from build123d import *

# Parameters (mm, degrees)
SKETCH1_R           = 6
SKETCH1_R_2         = 4.5
BOSS_EXTRUDE1_DEPTH = 0.5
CUT_EXTRUDE1_START  = -0.5
CUT_EXTRUDE1_DEPTH  = 0.5
FILLET1_R           = 1


with BuildPart() as part:
    # Sketch1 → Boss-Extrude1 (new body)
    with BuildSketch(Plane.XY):
        Circle(SKETCH1_R)
        Circle(SKETCH1_R_2, mode=Mode.SUBTRACT)
    extrude(amount=BOSS_EXTRUDE1_DEPTH)

    # Sketch2 → Cut-Extrude1 (cut)
    with BuildSketch(Plane.XY.offset(0.5).offset(CUT_EXTRUDE1_START)):
        with BuildLine():
            Line((5.637224766, 2.054676846), (4.227918574, 1.541007634))
            ThreePointArc((4.227918574, 1.541007634), (4.431457637, 0.782421375), (4.5, 0))
            ThreePointArc((4.5, 0), (4.431457637, -0.782421375), (4.227918574, -1.541007634))
            Line((4.227918574, -1.541007634), (5.637224766, -2.054676846))
            ThreePointArc((5.637224766, -2.054676846), (5.908610183, -1.0432285), (6, 0))
            ThreePointArc((6, 0), (5.908610183, 1.0432285), (5.637224766, 2.054676846))
        make_face()
    extrude(amount=CUT_EXTRUDE1_DEPTH, mode=Mode.SUBTRACT)

    # Fillet1
    # the kernel refuses this fillet: 1 mm, written as the material it takes off along each edge
    with BuildSketch(Plane(origin=(4.227918574, -1.541007634, -2.270817283), x_dir=(0.9395374609645726, -0.3424461409393371, 0), z_dir=(0, 0, 1))) as fillet1_piece_1:
        with BuildLine():
            CenterArc((0.908326913, -1), FILLET1_R, 90, 79.524318304)
            ThreePointArc((-0.075005253, -0.818181818), (-0.018790545, -0.410806303), (0, 0))
            Line((0, 0), (0.908326913, 0))
        make_face()
    extrude(amount=5.041634566, mode=Mode.SUBTRACT)
    with BuildSketch(Plane(origin=(5.637224766, -2.054676846, -3.01526886), x_dir=(-0.4351439810441928, -0.9003608808477915, 0), z_dir=(0, 0, 1))) as fillet1_piece_2:
        with BuildLine():
            CenterArc((1.105598582, -0.994936153), FILLET1_R, 84.231520484, 101.536959033)
            Line((0.110662429, -1.095445115), (0, 0))
            ThreePointArc((0, 0), (0.603053772, 0.030383082), (1.206107544, 0))
        make_face()
    extrude(amount=6.53053772, mode=Mode.SUBTRACT)
    with BuildSketch(Plane(origin=(4.227918574, 1.541007634, -2.270817283), x_dir=(0.9395374609645728, 0.3424461409393367, 0), z_dir=(0, 0, 1))) as fillet1_piece_3:
        with BuildLine():
            CenterArc((0.908326913, 1), FILLET1_R, 190.475681696, 79.524318304)
            ThreePointArc((-0.075005253, 0.818181818), (-0.018790545, 0.410806303), (0, 0))
            Line((0, 0), (0.908326913, 0))
        make_face()
    extrude(amount=5.041634566, mode=Mode.SUBTRACT)
    with BuildSketch(Plane(origin=(5.637224766, 2.054676846, -3.01526886), x_dir=(-0.43514398104419194, 0.9003608808477921, 0), z_dir=(0, 0, 1))) as fillet1_piece_4:
        with BuildLine():
            CenterArc((1.105598582, 0.994936153), FILLET1_R, 174.231520484, 101.536959033)
            Line((0.110662429, 1.095445115), (0, 0))
            ThreePointArc((0, 0), (0.603053772, -0.030383082), (1.206107544, 0))
        make_face()
    extrude(amount=6.53053772, mode=Mode.SUBTRACT)


solid = part.part
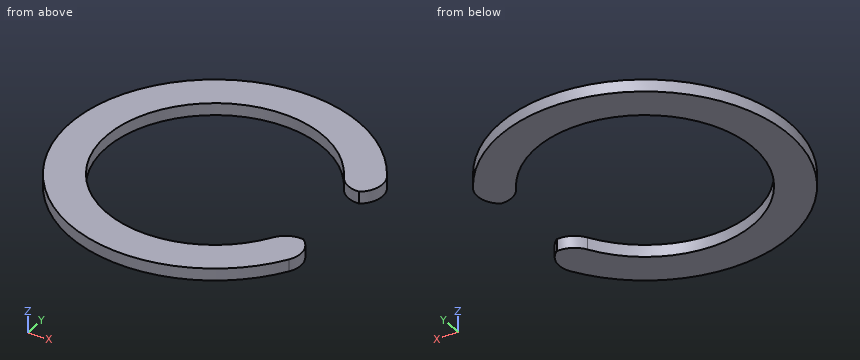
Source: CAD feature listing. Evaluate the final solid. Frame: model axes, mm. Give positions to 0.01 mm unless a question says otherwise; leave off trailing zeros. Write each loop counter-clockwise with the first axis right and the second up, starting at its lowest first coordinate (ties: lowest second). Pieces come first, ordered by that corner, then holes. Notation, with made-up numbers: (-13.5, -8.5) -> (9.5, -8.5) arc R21 ccw to (9.5, -4.5) -> close; hole circle Ø9 at (-20, -10.5). An arc over 180 degrees is marked (long way). Return JSON: item names as keys, results as strings. Group by question number.
1. Section D-D, the plane y = 0. Output: boundary loops of the cut face in (x, z).
2. Material intervals for line 1 (Y direction, x = 0, z = 0.15); line 2 (X direction, y = 0, z = 0.3); line 3 (Y direction, x = -1.25, z = 0.25), sorted ascending. Write a range as from..to.
3. Section C-C, the plane z = 0.35. Output: boundary loops of the cut face in (x, y).
4. Section A-A, the plane x = 0. Output: boundary loops of the cut face in (y, z), then the cut area to 3 significant figures.
5. Section B-B, the plane y = 4.25. Output: boundary loops of the cut face in (x, z), then the cut area to 3 significant figures.
Determined:
{
 "1": {"outline": "(-6, 0) -> (-4.5, 0) -> (-4.5, 0.5) -> (-6, 0.5) -> close"},
 "2": {"line 1": "y = -6..-4.5, 4.5..6", "line 2": "x = -6..-4.5", "line 3": "y = -5.87..-4.32, 4.32..5.87"},
 "3": {"outline": "(3.88, -2.28) arc R4.5 cw (long way) to (3.88, 2.28) arc R1 ccw to (4.83, 1.8) arc R1 ccw to (5.11, 3.14) arc R6 ccw (long way) to (5.11, -3.14) arc R1 ccw to (4.83, -1.8) arc R1 ccw to start"},
 "4": {"outline": "(-6, 0) -> (-4.5, 0) -> (-4.5, 0.5) -> (-6, 0.5) -> close; (4.5, 0) -> (6, 0) -> (6, 0.5) -> (4.5, 0.5) -> close", "area": "1.50 mm2"},
 "5": {"outline": "(-4.24, 0) -> (-1.48, 0) -> (-1.48, 0.5) -> (-4.24, 0.5) -> close; (1.48, 0) -> (4.24, 0) -> (4.24, 0.5) -> (1.48, 0.5) -> close", "area": "2.76 mm2"}
}
